from build123d import *

# Parameters (mm, degrees)
F0_W     = 149.702176
F0_H     = 151.402846
F1_DEPTH = 40
F2_W     = 151.402846
F2_H     = 115.410104
F3_DEPTH = 40
F4_W     = 152.249246
F4_H     = 115.410104
F5_DEPTH = 40


with BuildPart() as f1:
    # F0 (on Top) → F1 (new body)
    with BuildSketch(Plane.XY):
        Rectangle(F0_W, F0_H)
    extrude(amount=F1_DEPTH)

    # F2 (on face) → F3 (join)
    with BuildSketch(Plane.YZ.offset(74.851088)):
        Rectangle(F2_W, F2_H)
    extrude(amount=F3_DEPTH)

    # F4 (on face) → F5 (join)
    with BuildSketch(Plane(origin=(-74.851088, 0, 0), x_dir=(0, -1, 0), z_dir=(-1, 0, 0))):
        Rectangle(F4_W, F4_H)
    extrude(amount=F5_DEPTH)


solid = f1.part
The listing builds one solid part. Answer for the finished solid, in the listing's coordinates (mm). A direction names the side the tool comes from. Coordinates: 2 decimals unless noted, no trailing zeros. Order: outer loops, then holes, each group sorted by start corner. A loop starts at its lowest first (then second) coordinate and runs counter-clockwise, first axis right, second up. Notation, with made-up numbers: (21, -5) -> (46, -5) arc R7 cw to (46, 6) -> close; hole circle Ø1 at (22.25, 14.5). An arc over 180 degrees is marked (long way). Answer in a Markdown table with one row per item. Add a question column.
Item 1: Find section B-B (y = -38). Write down the section's boundary in (x, z), then the cut area to 3 significant figures.
Item 2: Which of the six approach directions +Z, -Z, +X, -X, +Y, -Y give full straight-line access (tool end or side, diameter ignored) to faces 1 (the face through (40, -75.701, 12)), 2 (the face through (74.851, -1, 49)), 3 (the face through (-95, 76.125, -1)), 4 (the face through (74.851, -1, -28)), 5 (the face through (40, 75.701, 12))?
Item 3: Find section A-A (z = -18.5). Write down the section's boundary in (x, y).
Item 4: Find the intervals of material crossed by L1, parallel to X at y = -7, z = 42; L2, parallel to Z at x = 65, y = 29; L3, parallel to Y at x = -27, z = 4.5, in increasing order. Write a range as from..to.
Item 5: Each of these flat-tipped pins is pushed along its axis until it touches: P1, Ø1, axis at x = 13.5, y = 26.5, coming from the +Z side; P2, Ø6, axis at x = -15.5, y = 46, coming from the -Z side. Where does it stop, or does it pass through?
Item 6: Find section C-C (x = -34.5). Write down the section's boundary in (y, z), then the cut area to 3 significant figures.
Result set:
| question | item | result |
|---|---|---|
| 1 | outline | (-114.85, -57.71) -> (-74.85, -57.71) -> (-74.85, 0) -> (74.85, 0) -> (74.85, -57.71) -> (114.85, -57.71) -> (114.85, 57.71) -> (74.85, 57.71) -> (74.85, 40) -> (-74.85, 40) -> (-74.85, 57.71) -> (-114.85, 57.71) -> close |
| 1 | area | 15,200 mm² |
| 2 | face 1 | +Z, -Z, +X, -Y |
| 2 | face 2 | +Z, +Y, -Y |
| 2 | face 3 | +Z, -Z, +X, -X, +Y |
| 2 | face 4 | -Z, +Y, -Y |
| 2 | face 5 | +Z, -Z, +X, +Y |
| 3 | outline | (-114.85, -76.12) -> (-74.85, -76.12) -> (-74.85, 76.12) -> (-114.85, 76.12) -> close; (74.85, -75.7) -> (114.85, -75.7) -> (114.85, 75.7) -> (74.85, 75.7) -> close |
| 4 | L1 | x = -114.85..-74.85, 74.85..114.85 |
| 4 | L2 | z = 0..40 |
| 4 | L3 | y = -75.7..75.7 |
| 5 | P1 | stops at z = 40 |
| 5 | P2 | stops at z = 0 |
| 6 | outline | (-75.7, 0) -> (75.7, 0) -> (75.7, 40) -> (-75.7, 40) -> close |
| 6 | area | 6,060 mm² |
